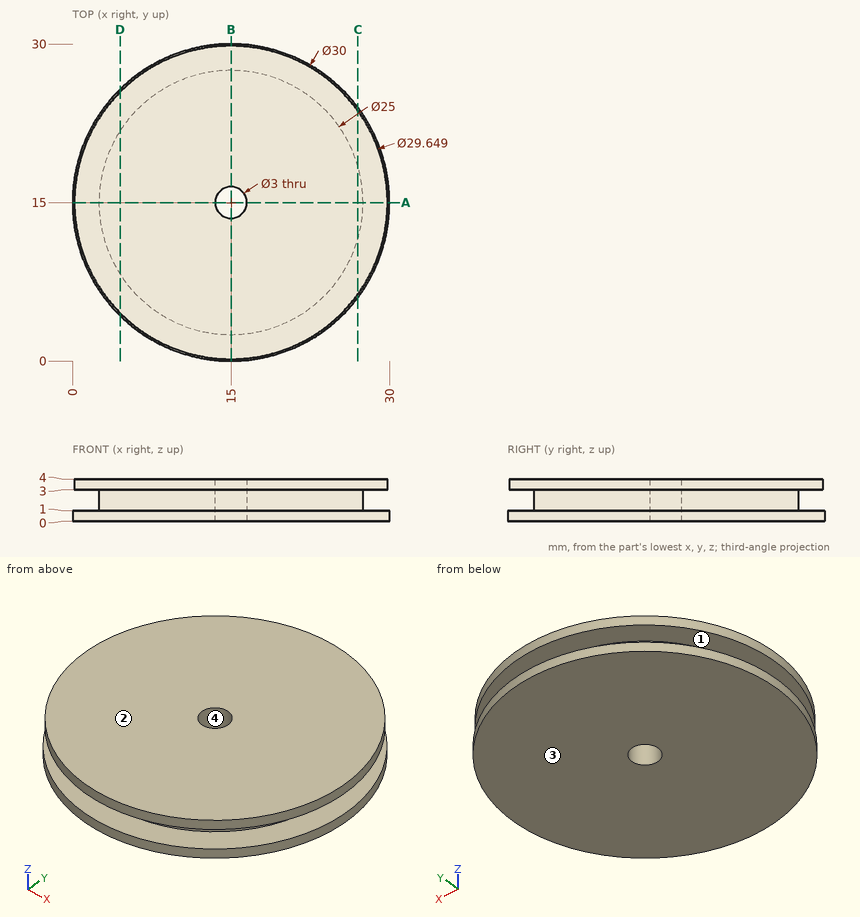
Print and shaded views of the part. All mm, measured from the part's lowest x, y and z. A direction names the side the tool comes from. Coordinates: 2 decimals unless noted, no trailing zeros. Order: outer loops, then holes, each group sorted by start corner. A loop starts at its lowest first (then second) coordinate and runs counter-clockwise, first axis right, second up. Notation, with made-up numbers: M 5,10.25 L 45,10.25 A26 cw 45,43.25 Z; hole C 59.5,-3.5 d10. An arc over 180 degrees is marked long. Write each question's results on one line, items separated by ' | '. Start each with the question number.
Q1. Which spindle directions (+Z, -Z, +X, -X, +Y, -Y) get a long thin tool onto all of the face, cutting with end or side? Do the marked faces 1 and 2. Say none if no direction does.
Q2. Cut at D-D (x = 4.5). List the corners of the cut face in (y, z).
Q3. Flat gauge pin, fed straight in: P1, Ø1.5, axis at y = 4.5, z = 2, coming from the +X side. Where does the tip first touch, or does it go through?
Q4. Drill centre lines: probe 1 along Z at (x, y) = (19.75, 1.5); probe 2 along Y at (x, z) = (15, 2.1); probe 3 along Y at (x, z) = (15, 3.1). Where is each one in solid material? Low to high. Write a range as from..to.
Q5. Pull direction X, two halves, no side cores. Call the marked faces 3 and 4: +X half, -X half, draft (parallel to the pull), parting line (faces both ways), or undercut.
Q6. Cut at A-A (y = 15). List the corners of the cut face in (x, z).
Q7. Cut at C-C (x = 27). List the corners of the cut face in (y, z).
Found:
1) face 1: none | face 2: +Z, +X, -X, +Y, -Y
2) outline: M 4.29,0 L 25.71,0 L 25.71,1 L 21.78,1 L 21.78,3 L 25.46,3 L 25.46,4 L 4.54,4 L 4.54,3 L 8.22,3 L 8.22,1 L 4.29,1 Z
3) P1: x = 22.82
4) probe 1: 0..1, 3..4 | probe 2: 2.5..13.5, 16.5..27.5 | probe 3: 0.18..13.5, 16.5..29.82
5) face 3: draft | face 4: undercut
6) outline: M 0,0 L 13.5,0 L 13.5,4 L 0.18,4 L 0.18,3 L 2.5,3 L 2.5,1 L 0,1 Z; M 16.5,0 L 30,0 L 30,1 L 27.5,1 L 27.5,3 L 29.82,3 L 29.82,4 L 16.5,4 Z
7) outline: M 6,0 L 24,0 L 24,1 L 18.5,1 L 18.5,3 L 23.7,3 L 23.7,4 L 6.3,4 L 6.3,3 L 11.5,3 L 11.5,1 L 6,1 Z
